Work out the finished part from the listing and answer in its coordinate system (mm). A direction names the side the tool comes from. Round coordinates to 2 decimals unless told otherwise and drop trailing zeros. Write each loop counter-clockwise with the first axis right and the second up, starting at its lowest first coordinate (ties: lowest second). Pieces come first, ordered by that corner, then holes. Notation, with made-up numbers: (-26, -33.75) - (-8, -33.75) arc R13 ccw to (-8, -16.75) - close; hole circle Ø11 at (11.5, 74). An arc over 180 degrees is marked (long way). Write item = value, one per line. Start each with the question number.
from build123d import *

# Parameters (mm, degrees)
F0_R      = 9.9
F0_R_2    = 7.9
F1_DEPTH  = 12
F3_DEPTH  = 12
F5_DEPTH  = 12.001
F6_W      = 2
F6_H      = 4.608413
F7_DEPTH  = 12.001
F8_W      = 2
F8_H      = 8
F9_DEPTH  = 12
F10_R     = 1.5
F11_DEPTH = 12.901
F13_DEPTH = 0.5


with BuildPart() as f1:
    # F0 (on Top) → F1 (new body)
    with BuildSketch(Plane.XY):
        Circle(F0_R)
        Circle(F0_R_2, mode=Mode.SUBTRACT)
    extrude(amount=F1_DEPTH)

    # F2 (on Top) → F3 (join)
    with BuildSketch(Plane.XY):
        Polygon((4, -9.055937), (0, -9.055937), (-4, -9.055937), (-4, -10.755937), (4, -10.755937), align=None)
    extrude(amount=F3_DEPTH)

    # F4 (on Top) → F5 (cut, through all)
    with BuildSketch(Plane.XY):
        Polygon((4, -9.055937), (2.5, -9.055937), (2.95, -10.755937), (4, -10.755937), align=None)
        Polygon((-2.95, -10.755937), (-2.5, -9.055937), (-4, -9.055937), (-4, -10.755937), align=None)
    extrude(amount=F5_DEPTH, mode=Mode.SUBTRACT)

    # F6 (on face) → F7 (cut, through all)
    with BuildSketch(Plane.XY.offset(12)):
        with Locations((0, 10.140659)):
            Rectangle(F6_W, F6_H)
    extrude(amount=-F7_DEPTH, mode=Mode.SUBTRACT)

    # F8 (on Top) → F9 (join)
    with BuildSketch(Plane.XY):
        with Locations((-2, 12.724238)):
            Rectangle(F8_W, F8_H)
        with Locations((2, 12.724238)):
            Rectangle(F8_W, F8_H)
    extrude(amount=F9_DEPTH)

    # F10 (on face) → F11 (cut, through all)
    with BuildSketch(Plane.YZ.offset(3)):
        with Locations((13.079374, 6)):
            Circle(F10_R)
    extrude(amount=-F11_DEPTH, mode=Mode.SUBTRACT)

    # F12 (on face) → F13 (cut)
    with BuildSketch(Plane(origin=(-3, 0, 0), x_dir=(0, -1, 0), z_dir=(-1, 0, 0))):
        Polygon((-13.104217, 8.944382), (-15.641705, 7.450677), (-15.616863, 4.506295), (-13.054532, 3.055618), (-10.517044, 4.549323), (-10.541886, 7.493705), align=None)
    extrude(amount=-F13_DEPTH, mode=Mode.SUBTRACT)


solid = f1.part
1. For a pull along Y with two mould halves and no side action, classify faces 1 (the face through (0, -10.756, 6)), 2 (the face through (1, 11, 6)), 3 (the face through (9.893, 0.367, 5.916)), 4 (the face through (-1.739, 14.465, 5.425)) as released by +Y, released by -Y, zero draft, split by the parting line, or undercut.
2. Find section C-C on z = 6. Give the vertices of the cut face in (x, y), plus the area to 3 significant figures.
3. Consider line 1 (X direction, y = 0, z = 8); line 2 (Y direction, x = -2, z = 5); line 3 (X direction, y = 9.5, z = 4.5). Determine where each line is inside the solid, lowest interval first.
4. Which of the six approach directions +Z, -Z, +X, -X, +Y, -Y give full straight-line access (tool end or side, diameter ignored) to faces 5 (the face through (-3, -9.056, 6)), 6 (the face through (-1, 11, 6)), 7 (the face through (3, 12.2, 4.6)), 8 (the face through (3, -9.056, 6)), 9 (the face through (-2.75, 11.81, 8.21))?
5. Each of these flat-tipped pins is pushed along its axis until it touches: pin 1 (2.5 mm diameter, centred on y = 13.08, z = 6, fed in from -X); pin 2 (2 mm diameter, centred on x = -4.5, z = 10, fed in from +Y); pin 3 (2 mm diameter, centred on y = 12, z = 3, fed in from +X); pin 4 (5 mm diameter, centred on y = 13.08, z = 6, fed in from -X). Where does it stop, or does it pass through?
6. Find section A-A on y = 0. Give the vertices of the cut face in (x, z).
7. Find section B-B on x = 2. Give the vertices of the cut face in (y, z), plus the area to 3 significant figures.
8. Find section D-D on z = 2.75. Give the vertices of the cut face in (x, y).
Answer key:
q1.face_1 = released by -Y
q1.face_2 = zero draft
q1.face_3 = split by the parting line
q1.face_4 = undercut
q2.outline = (-4, -9.06) - (-2.5, -9.06) - (-2.95, -10.76) - (2.95, -10.76) - (2.5, -9.06) - (4, -9.06) arc R9.9 ccw to (3, 9.43) - (3, 11.58) - (1, 11.58) - (1, 7.84) arc R7.9 cw (long way) to (-1, 7.84) - (-1, 11.58) - (-2.5, 11.58) - (-2.5, 10.53) - (-3, 10.53) - (-3, 9.43) arc R9.9 ccw to start; (-3, 15.63) - (-2.5, 15.63) - (-2.5, 14.58) - (-1, 14.58) - (-1, 16.72) - (-3, 16.72) - close; (1, 14.58) - (3, 14.58) - (3, 16.72) - (1, 16.72) - close
q2.area = 128 mm²
q3.line_1 = -9.9 to -7.9, 7.9 to 9.9
q3.line_2 = -10.76 to -7.64, 7.64 to 11.96, 14.2 to 16.72
q3.line_3 = -3 to -1, 1 to 3
q4.face_5 = +Z, -Z, -X
q4.face_6 = +Z, -Z, +Y
q4.face_7 = +Z, -Z, +X, +Y
q4.face_8 = +Z, -Z, +X
q4.face_9 = -X
q5.pin_1 = through
q5.pin_2 = 9.26
q5.pin_3 = 3
q5.pin_4 = -2.5
q6.outline = (-9.9, 0) - (-7.9, 0) - (-7.9, 12) - (-9.9, 12) - close; (7.9, 0) - (9.9, 0) - (9.9, 12) - (7.9, 12) - close
q7.outline = (-10.76, 0) - (-7.64, 0) - (-7.64, 12) - (-10.76, 12) - close; (7.64, 0) - (16.72, 0) - (16.72, 12) - (7.64, 12) - close; hole circle Ø3 at (13.08, 6)
q7.area = 139 mm²
q8.outline = (-4, -9.06) - (-2.5, -9.06) - (-2.95, -10.76) - (2.95, -10.76) - (2.5, -9.06) - (4, -9.06) arc R9.9 ccw to (3, 9.43) - (3, 16.72) - (1, 16.72) - (1, 7.84) arc R7.9 cw (long way) to (-1, 7.84) - (-1, 16.72) - (-3, 16.72) - (-3, 9.43) arc R9.9 ccw to start
